from build123d import *

# Parameters (mm, degrees)
SKETCH1_R               = 22.5
BOSS_EXTRUDE1_DEPTH     = 3
SKETCH2_R               = 5
BOSS_EXTRUDE2_DEPTH     = 70
SKETCH3_R               = 12
BOSS_EXTRUDE3_DEPTH     = 28
CUT_EXTRUDE1_DEPTH      = 80.633535649
CUT_EXTRUDE1_DEPTH_BACK = 80.633535649
SKETCH4_W               = 12.026752758
SKETCH4_H               = 20
FILLET1_R               = 6
CUT_EXTRUDE3_DEPTH      = 83.068568892
CUT_EXTRUDE3_DEPTH_BACK = 83.068568892
SKETCH6_R               = 4
SKETCH9_R               = 9
SKETCH9_R_2             = 4
BOSS_EXTRUDE4_DEPTH     = 12.5


with BuildPart() as part:
    # Sketch1 → Boss-Extrude1 (new body)
    with BuildSketch(Plane(origin=(0, 0, 0), x_dir=(1, 0, 0), z_dir=(0, 1, 0))):
        with Locations(Location((0, 0, 0), (0, 0, 270))):
            Circle(SKETCH1_R)
    extrude(amount=BOSS_EXTRUDE1_DEPTH)

    # Sketch2 → Boss-Extrude2 (add)
    with BuildSketch(Plane(origin=(0, 3, 0), x_dir=(1, 0, 0), z_dir=(0, 1, 0))):
        with Locations(Location((0, 0, 0), (0, 0, 270))):
            Circle(SKETCH2_R)
    extrude(amount=BOSS_EXTRUDE2_DEPTH)

    # Sketch3 → Boss-Extrude3 (add)
    with BuildSketch(Plane.XZ):
        with Locations(Location((0, 0, 0), (0, 0, 270))):
            Circle(SKETCH3_R)
    extrude(amount=BOSS_EXTRUDE3_DEPTH)

    # Sketch4 → Cut-Extrude1 (cut, two sides: drawn at the far end of the back side and taken through both)
    with BuildSketch(Plane.XY.offset(-CUT_EXTRUDE1_DEPTH_BACK)):
        with Locations((13.513376379, -18)):
            Rectangle(SKETCH4_W, SKETCH4_H)
        with Locations((-13.513376379, -18)):
            Rectangle(SKETCH4_W, SKETCH4_H)
    extrude(amount=CUT_EXTRUDE1_DEPTH + CUT_EXTRUDE1_DEPTH_BACK, mode=Mode.SUBTRACT)

    # Fillet1
    # the kernel refuses this fillet: 6 mm, written as the material it takes off along each edge
    with BuildSketch(Plane(origin=(0, -28, 0), x_dir=(0.9377485647369962, 0, -0.3473148849872455), z_dir=(-0.3473148849872455, 0, -0.9377485647369962))) as fillet1_piece_1:
        with BuildLine():
            CenterArc((12 - FILLET1_R, -FILLET1_R), FILLET1_R, 0, 90)
            Line((12 - FILLET1_R, 0), (12, 0))
            Line((12, 0), (12, -FILLET1_R))
        make_face()
    revolve(axis=Axis((0, -28, 0), (0, -1, 0)), revolution_arc=220.646338322, mode=Mode.SUBTRACT)
    with BuildSketch(Plane(origin=(0, -28, 0), x_dir=(0, 0, -1), z_dir=(-1, 0, 0))) as fillet1_piece_2:
        with BuildLine():
            CenterArc((12 - FILLET1_R, -FILLET1_R), FILLET1_R, 0, 90)
            Line((12 - FILLET1_R, 0), (12, 0))
            Line((12, 0), (12, -FILLET1_R))
        make_face()
    revolve(axis=Axis((0, -28, 0), (0, -1, 0)), revolution_arc=110.307225346, mode=Mode.SUBTRACT)
    with BuildSketch(Plane(origin=(0, -28, 0), x_dir=(-0.9378451764605575, 0, 0.34705392230842963), z_dir=(0.34705392230842963, 0, 0.9378451764605575))) as fillet1_piece_3:
        with BuildLine():
            CenterArc((12 - FILLET1_R, -FILLET1_R), FILLET1_R, 0, 90)
            Line((12 - FILLET1_R, 0), (12, 0))
            Line((12, 0), (12, -FILLET1_R))
        make_face()
    revolve(axis=Axis((0, -28, 0), (0, -1, 0)), revolution_arc=110.307225346, mode=Mode.SUBTRACT)

    # Sketch6 → Cut-Extrude3 (cut, two sides: drawn at the far end of the back side and taken through both)
    with BuildSketch(Plane(origin=(7.5, 0, 0), x_dir=(0, 0, -1), z_dir=(1, 0, 0)).offset(-CUT_EXTRUDE3_DEPTH_BACK)):
        with Locations(Location((0, -18, 0), (0, 0, 90))):
            Circle(SKETCH6_R)
    extrude(amount=CUT_EXTRUDE3_DEPTH + CUT_EXTRUDE3_DEPTH_BACK, mode=Mode.SUBTRACT)

    # Sketch9 → Boss-Extrude4 (add, symmetric)
    with BuildSketch(Plane(origin=(0, 0, 0), x_dir=(0, 0, -1), z_dir=(1, 0, 0))):
        with Locations(Location((0, -17.234671311, 0), (0, 0, 90))):
            Circle(SKETCH9_R)
        with Locations((0, -17.234671311)):
            Circle(SKETCH9_R_2, mode=Mode.SUBTRACT)
    extrude(amount=BOSS_EXTRUDE4_DEPTH, both=True)


solid = part.part
Build history of the part. All positions in model axes, mm. A direction names the side the tool comes from. Round coordinates to 2 decimals unless told otherwise and drop trailing zeros. Loops run counter-clockwise (first coordinate to the right, second up) from the corner with the lowest first, then second, coordinate; pieces in that order, holes last. Notation, with made-up numbers: (30, 22.25) -> (56, 22.25) arc R32 ccw to (56, 48.25) -> close; hole circle Ø7 at (-18, -21). An arc over 180 degrees is marked (long way). One line per item, written item: value. Start each with the question number.
Q1. Cut at C-C on x = 15.5. List the corners of the cut face in (y, z), plus the area to 3 significant figures.
Q2. Cut at A-A on y = -11.5. List the corners of the cut face in (x, z).
Q3. Drop flat-ended pins along their axis: pin 1 Ø2 at (x, z) = (-7, -17.5) entering from +Y; pin 2 Ø9 at (y, z) = (-15.5, -4.5) entering from +X; pin 3 Ø9.5 at (y, z) = (-20, -3) entering from -X. Give the stop position or say it passes through.
Q4. Probe line 1 along Y through (x, z) = (1.5, 0); line 2 along Y through (x, z) = (-6, 0); line 3 along Y through (x, z) = (17, 12). List the from-to ranges inside material, lowest first.
Q5. Cut at D-D on y = 59. List the corners of the cut face in (x, z), plus the area to 3 significant figures.
Q6. Two-plate mould, pull along Y, no slides. Class faces 1 (the face through (5.3, 3, -0.3)), 2 (the face through (-12.5, -15, -4)), 3 (the face through (-10.646, -5.957, -5.537)), 4 (the face through (0, -28, 0)): released by +Y, released by -Y, zero draft, split by the parting line, or undercut.
Q7. 3-axis set-ups, long thin cutter, end or side, ignore diameter. For faces 5 (the face through (-7.5, -13.8, -0.3)), 6 (the face through (7.5, -13.8, -0.3)), 7 (the face through (0, -14, 0)), 8 (the face through (9, -8, 0)), 9 (the face through (-4.88, 37.51, -1.08)): which of +Z, -Z, +X, -X, +Y, -Y reach the whole face in a straight line?
Q8. Cut at B-B on z = 16. List the corners of the cut face in (x, y), plus the area to 3 significant figures.
Computed:
1. outline: (0, -16.31) -> (3, -16.31) -> (3, 16.31) -> (0, 16.31) -> close
1. area: 97.9 mm²
2. outline: (-12.5, -6.94) -> (-7.5, -6.94) -> (-7.5, -9.37) arc R12 ccw to (7.5, -9.37) -> (7.5, -6.94) -> (12.5, -6.94) -> (12.5, 6.94) -> (7.5, 6.94) -> (7.5, 9.37) arc R12 ccw to (-7.5, 9.37) -> (-7.5, 6.94) -> (-12.5, 6.94) -> close
3. pin 1: y = 3
3. pin 2: x = 12.5
3. pin 3: x = -12.5
4. line 1: -28 to -21.23, -14 to 73
4. line 2: -28 to -21.23, -14 to 3
4. line 3: 0 to 3
5. outline: circle Ø10 at (0, 0)
5. area: 78.5 mm²
6. face 1: released by +Y
6. face 2: zero draft
6. face 3: undercut
6. face 4: released by -Y
7. face 5: -X
7. face 6: +X
7. face 7: +X, -X
7. face 8: +Z, -Z, +X
7. face 9: +Y
8. outline: (-15.82, 0) -> (15.82, 0) -> (15.82, 3) -> (-15.82, 3) -> close
8. area: 94.9 mm²
